Here's how the part is built. I have some questions about the finished solid (model axes, mm). Round coordinates to 2 decimals unless told otherwise and drop trailing zeros. Order: outer loops, then holes, each group sorted by start corner. A loop starts at its lowest first (then second) coordinate and runs counter-clockwise, first axis right, second up. Notation, with made-up numbers: (78.5, -21.75) -> (88.5, -21.75) arc R20 ccw to (88.5, -1.75) -> close; hole circle Ø5 at (59.5, 87). An arc over 180 degrees is marked (long way). Answer in a Markdown table with one row per item.
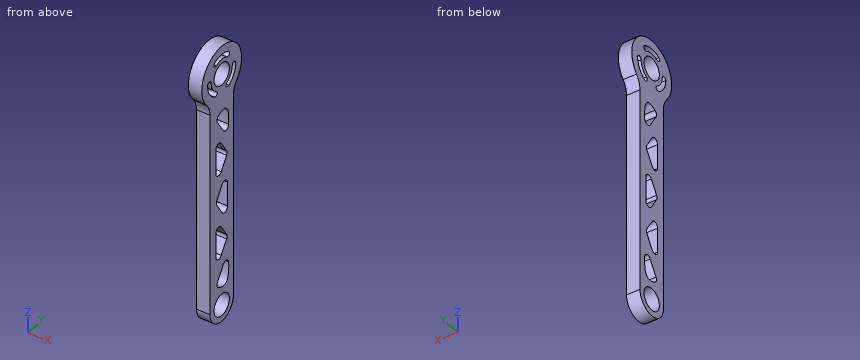
```python
from build123d import *

# Parameters (mm, degrees)
SKETCH_1_R      = 6.55
EXTRUDE_1_DEPTH = 8


with BuildPart() as part:
    # 草图1 → 凸台-拉伸1 (new body)
    with BuildSketch(Plane(origin=(-4, 0, 0), x_dir=(0, -1, 0), z_dir=(-1, 0, 0))):
        with BuildLine():
            Line((-10, -18.894443628), (-10, -140))
            ThreePointArc((-10, -140), (0, -150), (10, -140))
            Line((10, -140), (10, -18.894443628))
            ThreePointArc((10, -18.894443628), (10.74741409, -14.725593625), (12.896551724, -11.076053161))
            ThreePointArc((12.896551724, -11.076053161), (0, 17), (-12.896551724, -11.076053161))
            ThreePointArc((-12.896551724, -11.076053161), (-10.74741409, -14.725593625), (-10, -18.894443628))
        make_face()
        with Locations((0, -140)):
            Circle(SKETCH_1_R, mode=Mode.SUBTRACT)
        Circle(SKETCH_1_R, mode=Mode.SUBTRACT)
        with BuildLine():
            Line((-4.168179012, -99.797532142), (0.381550311, -92.536811957))
            ThreePointArc((0.381550311, -92.536811957), (3.190606899, -91.461560083), (5, -93.864279815))
            Line((5, -93.864279815), (5, -108.385720185))
            ThreePointArc((5, -108.385720185), (3.190606899, -110.788439917), (0.381550311, -109.713188043))
            Line((0.381550311, -109.713188043), (-4.168179012, -102.452467858))
            ThreePointArc((-4.168179012, -102.452467858), (-4.549729323, -101.125), (-4.168179012, -99.797532142))
        make_face(mode=Mode.SUBTRACT)
        with BuildLine():
            Line((-1.347932676, -116.369603301), (3.683273316, -124.398691695))
            ThreePointArc((3.683273316, -124.398691695), (3.98786354, -126.341689874), (2.792876182, -127.903746961))
            add(Edge.make_bspline(
                [(2.792876182, -127.903746961), (-2.877603269, -131.101619406), (-5.985402229, -127.808170374), (-6.076762251, -119.793304589), (-5.963124704, -117.569487096)],
                knots=[0.005408839, 0.005408839, 0.005408839, 0.005408839, 0.693539789, 0.980498212, 0.980498212, 0.980498212, 0.980498212], degree=3))
            ThreePointArc((-5.963124704, -117.569487096), (-4.09543452, -115.277506448), (-1.347932676, -116.369603301))
        make_face(mode=Mode.SUBTRACT)
        with BuildLine():
            Line((0.381550311, -58.963188043), (-4.168179012, -51.702467858))
            ThreePointArc((-4.168179012, -51.702467858), (-4.549729323, -50.375), (-4.168179012, -49.047532142))
            Line((-4.168179012, -49.047532142), (0.381550311, -41.786811957))
            ThreePointArc((0.381550311, -41.786811957), (3.190606899, -40.711560083), (5, -43.114279815))
            Line((5, -43.114279815), (5, -57.635720185))
            ThreePointArc((5, -57.635720185), (3.190606899, -60.038439917), (0.381550311, -58.963188043))
        make_face(mode=Mode.SUBTRACT)
        with BuildLine():
            Line((3.683273317, -27.101308304), (-1.347932676, -35.130396699))
            ThreePointArc((-1.347932676, -35.130396699), (-4.095434519, -36.222493552), (-5.963124704, -33.930512906))
            add(Edge.make_bspline(
                [(-5.963124704, -33.930512906), (-6.076762251, -31.706695412), (-5.98540223, -23.691829624), (-2.877603269, -20.398380591), (2.792876182, -23.596253037)],
                knots=[0.005408839, 0.005408839, 0.005408839, 0.005408839, 0.292367263, 0.980498213, 0.980498213, 0.980498213, 0.980498213], degree=3))
            ThreePointArc((2.792876182, -23.596253037), (3.987863541, -25.158310124), (3.683273317, -27.101308304))
        make_face(mode=Mode.SUBTRACT)
        with BuildLine():
            Line((4.168179012, -77.077467858), (-0.381550311, -84.338188043))
            ThreePointArc((-0.381550311, -84.338188043), (-3.190606899, -85.413439917), (-5, -83.010720185))
            Line((-5, -83.010720185), (-5, -68.489279815))
            ThreePointArc((-5, -68.489279815), (-3.190606899, -66.086560083), (-0.381550311, -67.161811957))
            Line((-0.381550311, -67.161811957), (4.168179012, -74.422532142))
            ThreePointArc((4.168179012, -74.422532142), (4.549729323, -75.75), (4.168179012, -77.077467858))
        make_face(mode=Mode.SUBTRACT)
        with BuildLine():
            ThreePointArc((-4.5, 7.794228634), (-6.549038106, 8.34326674), (-6, 10.392304845))
            ThreePointArc((-6, 10.392304845), (0, 12), (6, 10.392304845))
            ThreePointArc((6, 10.392304845), (6.549038106, 8.34326674), (4.5, 7.794228634))
            ThreePointArc((4.5, 7.794228634), (0, 9), (-4.5, 7.794228634))
        make_face(mode=Mode.SUBTRACT)
        with BuildLine():
            ThreePointArc((9, 0), (10.5, 1.5), (12, 0))
            ThreePointArc((12, 0), (10.392304845, -6), (6, -10.392304845))
            ThreePointArc((6, -10.392304845), (3.950961894, -9.84326674), (4.5, -7.794228634))
            ThreePointArc((4.5, -7.794228634), (7.794228634, -4.5), (9, 0))
        make_face(mode=Mode.SUBTRACT)
        with BuildLine():
            ThreePointArc((-4.5, -7.794228634), (-3.950961894, -9.84326674), (-6, -10.392304845))
            ThreePointArc((-6, -10.392304845), (-10.392304845, -6), (-12, 0))
            ThreePointArc((-12, 0), (-10.5, 1.5), (-9, 0))
            ThreePointArc((-9, 0), (-7.794228634, -4.5), (-4.5, -7.794228634))
        make_face(mode=Mode.SUBTRACT)
    extrude(amount=-EXTRUDE_1_DEPTH)


solid = part.part
```
1. Please list where these lines run through material, in increasing order: line 1 along Y through (x, z) = (-1, -5.5); line 2 along Y through (x, z) = (-0.5, -101); line 3 along Y through (x, z) = (-1.25, -140.5).
Numbers:
| item | result |
|---|---|
| line 1 | y = -16.09 to -10.67, -7.12 to -3.56, 3.56 to 7.12, 10.67 to 16.09 |
| line 2 | y = -10 to -5, 4.55 to 10 |
| line 3 | y = -9.99 to -6.53, 6.53 to 9.99 |
2. For pin 1 Ø1.5 at (x, z) = (3, -103) entering from -Y; pin 2 Ø17 at (y, z) = (0, -140) entering from +X; pin 3 Ø1 at (x, z) = (-1, -8) entering from +Y; pin 4 Ø2.5 at (x, z) = (-0.5, -51) entering from +Y, each with a flat end and sliding along its axis, tell me the tip position at first contact or that it passes through.
Numbers:
| item | result |
|---|---|
| pin 1 | stops at y = -10 |
| pin 2 | stops at x = 4 |
| pin 3 | stops at y = 15.26 |
| pin 4 | stops at y = 10 |
3. Suppose I cut it at A-A on x = -2.5. State how many separate pieces and enclosed holes the cut face has, then the cut area to 3 significant figures.
Numbers:
| item | result |
|---|---|
| separate pieces | 1 |
| enclosed holes | 10 |
| area | 2,570 mm2 |
4. Suppose I cut it at B-B on z = -64. Write out the boundary of the cut face in (x, y), then the cut area to 3 significant figures.
Numbers:
| item | result |
|---|---|
| outline | (-4, -10) -> (4, -10) -> (4, 10) -> (-4, 10) -> close |
| area | 160 mm2 |
